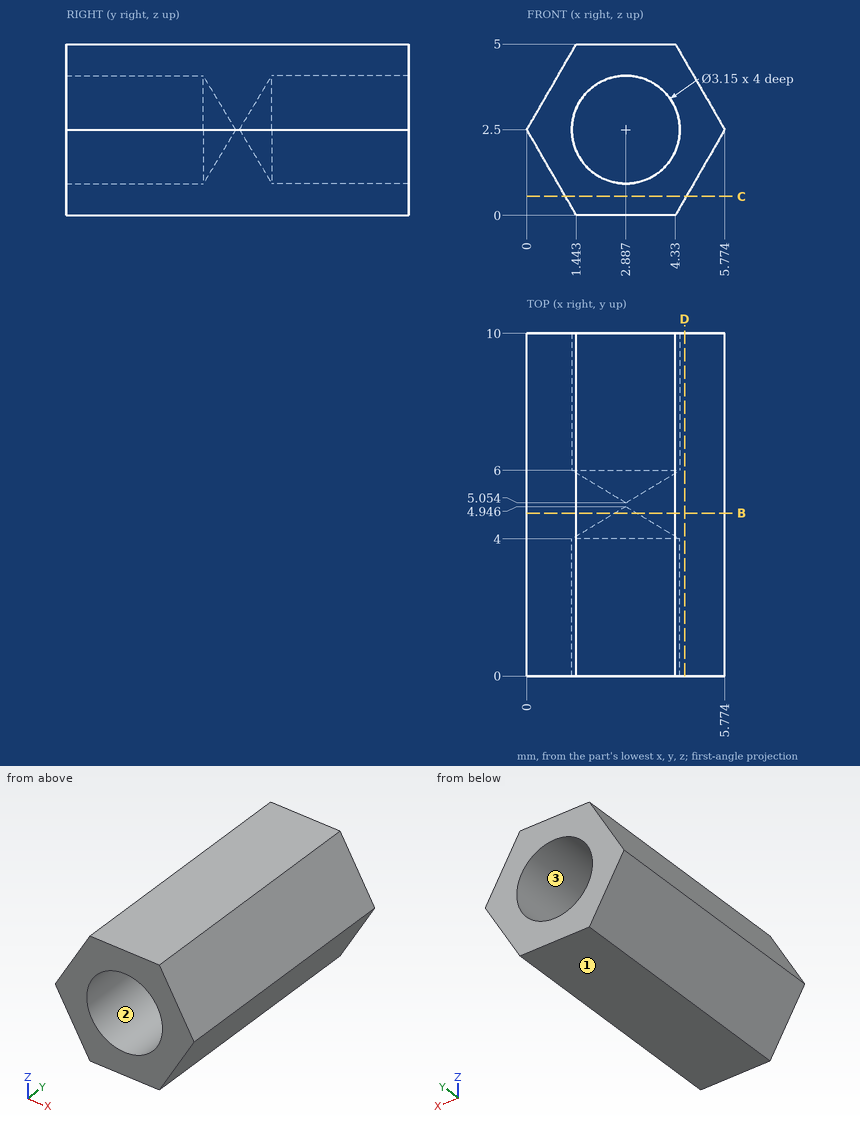
Can you work these out from the drawing? Everything is in mm from the part's minimum corner. A direction names the side the tool comes from. Give positions to 0.01 mm unless a question says otherwise; leave off trailing zeros. Order: outer loops, then holes, each group sorted by start corner. A loop starts at its lowest first (then second) coordinate and runs counter-clockwise, first axis right, second up. Notation, with made-up numbers: M 21,7 L 39,7 A17 ccw 39,21 Z; hole C -1,-17 d2. An arc over 180 degrees is marked long. Use a Markdown table: item, result. Add a question column.
Item 1: Suppose I cut it at D-D (x = 4.6). List the corners of the cut face in (y, z) for me.
Item 2: If I drill on L1, parallel to X at y = 2.5, z = 2.65 (1 decimal); L2, parallel to Z at x = 3.4, y = 8.25; L3, parallel to Z at x = 2.8, y = 3.5, over which ranges is the centre line in solid material (lowest first)? Write a range as [from, to].
Item 3: For the marked faces 1, 2 and 3, which set-ups out of +Z, -Z, +X, -X, +Y, -Y let a thin tool reach every point of the face, with its end or its side?
Item 4: Suppose I cut it at B-B (y = 4.75). List the corners of the cut face in (x, z) for me.
Item 5: Will this pin go through, and if not, where does the flat tip stop? pin 1 (1 mm diameter, centred on y = 6, z = 4.5, fed in from -X) (1 decimal).
Item 6: Suppose I cut it at C-C (z = 0.55). List the corners of the cut face in (x, y) for me (1 decimal), then the cut area to 3 significant figures.
Answer sheet:
| question | item | result |
|---|---|---|
| 1 | outline | M 0,0.47 L 10,0.47 L 10,4.53 L 0,4.53 Z |
| 2 | L1 | x = [0.1, 1.3], [4.5, 5.7] |
| 2 | L2 | z = [0, 1.01], [3.99, 5] |
| 2 | L3 | z = [0, 0.93], [4.07, 5] |
| 3 | face 1 | -Z, +X, -X, +Y, -Y |
| 3 | face 2 | -Y |
| 3 | face 3 | +Y |
| 4 | outline | M 0,2.5 L 1.44,0 L 4.33,0 L 5.77,2.5 L 4.33,5 L 1.44,5 Z; hole C 2.89,2.5 d0.65 |
| 5 | pin 1 | stops at x = 0.9 |
| 6 | outline | M 1.1,0 L 4.6,0 L 4.6,10 L 1.1,10 Z |
| 6 | area | 35.2 mm² |
